```python
from build123d import *

# Parameters (mm, degrees)
SKETCH1_W           = 59.2
SKETCH1_H           = 29.2
BOSS_EXTRUDE1_DEPTH = 1
SKETCH2_W           = 50.15
SKETCH2_H           = 25.3
CUT_EXTRUDE1_DEPTH  = 0.2
CUT_EXTRUDE2_DEPTH  = 42.590864381
SKETCH4_W           = 13.88
SKETCH4_H           = 0.707068884
BOSS_EXTRUDE2_DEPTH = 4.5


with BuildPart() as part:
    # Sketch1 → Boss-Extrude1 (new body)
    with BuildSketch(Plane(origin=(0, 0, 0), x_dir=(1, 0, 0), z_dir=(0, 1, 0))):
        Rectangle(SKETCH1_W, SKETCH1_H)
    extrude(amount=BOSS_EXTRUDE1_DEPTH)

    # Sketch2 → Cut-Extrude1 (cut)
    with BuildSketch(Plane(origin=(0, 1, 0), x_dir=(1, 0, 0), z_dir=(0, 1, 0))):
        with Locations((2.625, 0)):
            Rectangle(SKETCH2_W, SKETCH2_H)
    extrude(amount=-CUT_EXTRUDE1_DEPTH, mode=Mode.SUBTRACT)

    # Sketch3 → Cut-Extrude2 (cut, through all)
    with BuildSketch(Plane.XY.offset(14.6)):
        Polygon((-29.6, 0.5), (-25.80413761, 0.5), (-25.30413761, 1), (-29.6, 1), align=None)
    extrude(amount=-CUT_EXTRUDE2_DEPTH, mode=Mode.SUBTRACT)

    # Sketch4 → Boss-Extrude2 (add)
    with BuildSketch(Plane.ZY.offset(29.6)):
        with Locations((-0.89, 0.646465558)):
            Rectangle(SKETCH4_W, SKETCH4_H)
    extrude(amount=-BOSS_EXTRUDE2_DEPTH)


solid = part.part
```
The listing builds one solid part. Answer for the finished solid, in the listing's coordinates (mm). A direction names the side the tool comes from. Give positions to 0.01 mm unless a question says otherwise; leave off trailing zeros. Order: outer loops, then holes, each group sorted by start corner. A loop starts at its lowest first (then second) coordinate and runs counter-clockwise, first axis right, second up. Notation, with made-up numbers: (12, 79.5) -> (51, 79.5) arc R27 ccw to (51, 114.5) -> close; hole circle Ø5 at (52, 71.25). An arc over 180 degrees is marked (long way). One line per item, written item: value.
1) Find section B-B, the plane x = -13.5. Determine the outline of the cut face in (y, z), plus the area to 3 significant figures.
Reported:
outline: (0, -14.6) -> (1, -14.6) -> (1, -12.65) -> (0.8, -12.65) -> (0.8, 12.65) -> (1, 12.65) -> (1, 14.6) -> (0, 14.6) -> close
area: 24.1 mm^2
2) Find the intervals of material crossed by line 1 (Z direction, x = 19, y = 0.95); line 2 (Y direction, x = -27, z = -9.25); line 3 (Y direction, x = 15, z = 7.5), in increasing order.
Reported:
line 1: z = -14.6 to -12.65, 12.65 to 14.6
line 2: y = 0 to 0.5
line 3: y = 0 to 0.8
3) A tool of negligible diameter and unlimited length cuts with its end or side. For faces 1 (the flat face through (-28, 0.5, 10)), 2 (the flat face through (-29.6, 0.4, 0.2)), 3 (the flat face through (-28, 0.5, -11)), from which of +Z, -Z, +X, -X, +Y, -Y can it reach the whole face along a straight path? Write none if from no direction.
Reported:
face 1: +Z, -X, +Y
face 2: +Z, -Z, -X, +Y, -Y
face 3: -Z, -X, +Y
4) Flat-ended cylindrical pins translate along their axes: P1, Ø2, axis at x = 5.5, z = 9.5, coming from the -Y side; P2, Ø7.5, axis at x = 6, z = 0.5, coming from the +Y side; P3, Ø1.9, axis at x = -28, z = 11.5, coming from the +Y side. Find the tip coordinate at first contact, or state that the pin passes through.
Reported:
P1: stops at y = 0
P2: stops at y = 0.8
P3: stops at y = 0.5
5) Determine the mould class of faces 4 (the flat face through (-5, 1, -13)), 5 (the flat face through (2, 0.8, 0)), 6 (the flat face through (-0.4, 0.5, 14.6)) for opening direction Z: pulls with the +Z half, pulls with the -Z half, needs draft (parallel to the pull), parting line crosses it, or undercut.
Reported:
face 4: needs draft
face 5: undercut
face 6: pulls with the +Z half
6) Find section A-A, the plane z = 4. Determine the outline of the cut face in (x, y), plus the area to 3 significant figures.
Reported:
outline: (-29.6, 0) -> (29.6, 0) -> (29.6, 1) -> (27.7, 1) -> (27.7, 0.8) -> (-22.45, 0.8) -> (-22.45, 1) -> (-29.6, 1) -> close
area: 49.2 mm^2
